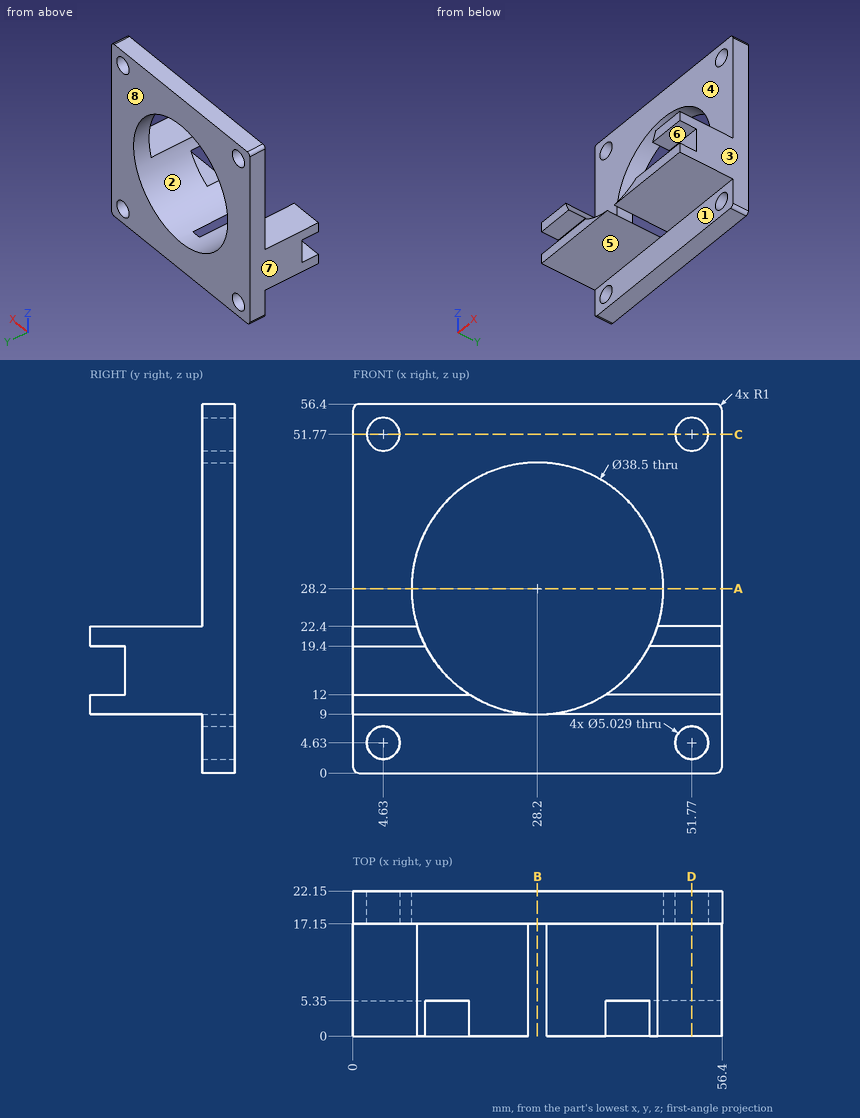
Here's the drawing with two shaded views (mm, measured from the low corner). I have some questions. A direction names the side the tool comes from. Give positions to 0.01 mm unless a question says otherwise; leave off trailing zeros. Order: outer loops, then holes, each group sorted by start corner. A loop starts at its lowest first (then second) coordinate and runs counter-clockwise, first axis right, second up. Notation, with made-up numbers: (76.5, 10.5) -> (134.5, 10.5) arc R26 ccw to (134.5, 26.5) -> close; hole circle Ø7 at (-27.5, -17). An arc over 180 degrees is marked (long way). Use a Markdown table: item, result. Add a question column.
Item 1: Imagine slicing it at A-A on z = 28.2. Please give me the cut outline in (x, y).
Item 2: For the marked faces 4, 5, 6, 7 and 8, which set-ups out of +Z, -Z, +X, -X, +Y, -Y let a thin tool reach every point of the face, with its end or its side?
Item 3: If we mould it in two halves opening along X, with no side actions, what happens to the marked faces 1, 2 and 3? For each: pulls with the +X half, pulls with the -X half, needs draft (parallel to the pull), parting line crosses it, or undercut.
Item 4: I need wall thicknesses on line 1 (X direction, y = 20.25, z = 51.77); line 2 (Z direction, x = 9, y = 3). Which ranges of each line are inside material? Lowest first, please.
Item 5: Imagine slicing it at D-D on x = 51.77. Please give me the cut outline in (y, z), plus the area to 3 significant figures.
Item 6: Imagine slicing it at C-C on z = 51.77. Please give me the cut outline in (x, y).
Item 7: Will these pins go through, and if not, where does the flat tip stop? pin 1 (6 mm diameter, centred on x = 35.5, z = 46, fed in from -Y); pin 2 (4.5 mm diameter, centred on x = 6, y = 2, fed in from +Z); pin 3 (1 mm diameter, centred on y = 15.5, z = 35.5, fed in from -X); pin 4 (1.6 mm diameter, centred on x = 5, y = 2, fed in from -Z).
Item 8: Imagine slicing it at B-B on x = 28.2. Please give me the cut outline in (y, z), plus the area to 3 significant figures.
Data:
| question | item | result |
|---|---|---|
| 1 | outline | (0, 17.15) -> (8.95, 17.15) -> (8.95, 22.15) -> (0, 22.15) -> close; (47.45, 17.15) -> (56.4, 17.15) -> (56.4, 22.15) -> (47.45, 22.15) -> close |
| 2 | face 4 | +Z, +X, -X, -Y |
| 2 | face 5 | -Z, +X, -X, -Y |
| 2 | face 6 | +X, -X, -Y |
| 2 | face 7 | +Z, -Z, -X, +Y, -Y |
| 2 | face 8 | +Z, -Z, +X, -X, +Y |
| 3 | face 1 | needs draft |
| 3 | face 2 | undercut |
| 3 | face 3 | pulls with the +X half |
| 4 | line 1 | x = 0 to 2.12, 7.14 to 49.26, 54.28 to 56.4 |
| 4 | line 2 | z = 9 to 12, 19.4 to 22.4 |
| 5 | outline | (0, 9) -> (17.15, 9) -> (17.15, 7.14) -> (22.15, 7.14) -> (22.15, 49.26) -> (17.15, 49.26) -> (17.15, 22.4) -> (0, 22.4) -> (0, 19.4) -> (5.35, 19.4) -> (5.35, 12) -> (0, 12) -> close; (17.15, 0) -> (22.15, 0) -> (22.15, 2.12) -> (17.15, 2.12) -> close; (17.15, 54.28) -> (22.15, 54.28) -> (22.15, 56.4) -> (17.15, 56.4) -> close |
| 5 | area | 422 mm² |
| 6 | outline | (0, 17.15) -> (2.12, 17.15) -> (2.12, 22.15) -> (0, 22.15) -> close; (7.14, 17.15) -> (49.26, 17.15) -> (49.26, 22.15) -> (7.14, 22.15) -> close; (54.28, 17.15) -> (56.4, 17.15) -> (56.4, 22.15) -> (54.28, 22.15) -> close |
| 7 | pin 1 | stops at y = 17.15 |
| 7 | pin 2 | stops at z = 22.4 |
| 7 | pin 3 | passes through |
| 7 | pin 4 | stops at z = 9 |
| 8 | outline | (17.15, 0) -> (22.15, 0) -> (22.15, 8.95) -> (17.15, 8.95) -> close; (17.15, 47.45) -> (22.15, 47.45) -> (22.15, 56.4) -> (17.15, 56.4) -> close |
| 8 | area | 89.5 mm² |
